Read the model definition and answer for the solid it produces. Units are mm, in the model's axes. Face numbers are marked on the shaded views. Round coordinates to 2 decimals unless told otherwise and drop trailing zeros. Loops run counter-clockwise (first coordinate to the right, second up) from the corner with the lowest first, then second, coordinate; pieces in that order, holes last. Notation, with made-up numbers: (-21, 64) - (25, 64) arc R22 cw to (25, 90) - close; hole circle Ø11 at (37.5, 41). An arc over 180 degrees is marked (long way). Answer as CSV lines item,"result".
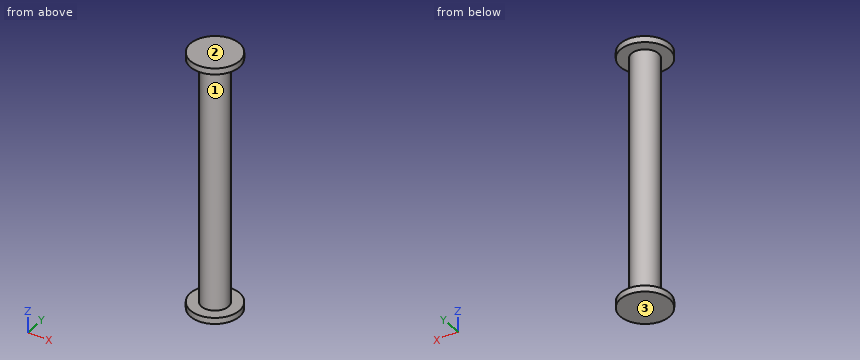
```python
from build123d import *

# Parameters (mm, degrees)
SKETCH1_R           = 2.2
BOSS_EXTRUDE1_DEPTH = 40
SKETCH2_R           = 4
BOSS_EXTRUDE2_DEPTH = 1
SKETCH3_R           = 4
BOSS_EXTRUDE3_DEPTH = 1


with BuildPart() as part:
    # Sketch1 → Boss-Extrude1 (new body)
    with BuildSketch(Plane.XY):
        with Locations((-44.111688034, 4.888301887)):
            Circle(SKETCH1_R)
    extrude(amount=-BOSS_EXTRUDE1_DEPTH)

    # Sketch2 → Boss-Extrude2 (add)
    with BuildSketch(Plane.XY):
        with Locations((-44.111688034, 4.888301887)):
            Circle(SKETCH2_R)
    extrude(amount=BOSS_EXTRUDE2_DEPTH)

    # Sketch3 → Boss-Extrude3 (add)
    with BuildSketch(Plane(origin=(0, 0, -40), x_dir=(-1, 0, 0), z_dir=(0, 0, -1))):
        with Locations((44.111688034, 4.888301887)):
            Circle(SKETCH3_R)
    extrude(amount=BOSS_EXTRUDE3_DEPTH)


solid = part.part
```
1) Each of these flat-tipped pins is pushed along its axis until it touches: P1, Ø2, axis at x = -46, z = -22.5, coming from the +Y side; P2, Ø3, axis at y = 4.5, z = -32.5, coming from the +X side; P3, Ø3, axis at y = 2.5, z = -27, coming from the -X side. Where does it stop, or does it pass through?
Entries:
P1,"stops at y = 6.9"
P2,"stops at x = -41.91"
P3,"stops at x = -46.12"
2) A cutting plane is placed at D-D, the plane x = -43.75. Determine the outline of the cut face in (y, z).
Entries:
outline,"(0.9, -41) - (8.87, -41) - (8.87, -40) - (7.06, -40) - (7.06, 0) - (8.87, 0) - (8.87, 1) - (0.9, 1) - (0.9, 0) - (2.72, 0) - (2.72, -40) - (0.9, -40) - close"
3) A cutting plane is placed at C-C, the plane y = 6.25. Determine the outline of the cut face in (x, z), plus the area to 3 significant figures.
Entries:
outline,"(-47.87, -41) - (-40.35, -41) - (-40.35, -40) - (-42.38, -40) - (-42.38, 0) - (-40.35, 0) - (-40.35, 1) - (-47.87, 1) - (-47.87, 0) - (-45.84, 0) - (-45.84, -40) - (-47.87, -40) - close"
area,"153 mm^2"
4) A cutting plane is placed at A-A, the plane x = -46.75. Determine the outline of the cut face in (y, z).
Entries:
outline,"(1.88, -41) - (7.89, -41) - (7.89, -40) - (1.88, -40) - close; (1.88, 0) - (7.89, 0) - (7.89, 1) - (1.88, 1) - close"
5) A cutting plane is placed at B-B, the plane y = 1.5. Determine the outline of the cut face in (x, z), plus the area to 3 significant figures.
Entries:
outline,"(-46.24, -41) - (-41.99, -41) - (-41.99, -40) - (-46.24, -40) - close; (-46.24, 0) - (-41.99, 0) - (-41.99, 1) - (-46.24, 1) - close"
area,"8.50 mm^2"
6) Find the intervals of material crossed by line 1 (Z direction, x = -45, y = 7.25); line 2 (X direction, y = 5, z = -14.5); line 3 (Y direction, x = -43.5, z = -18), in increasing order.
Entries:
line 1,"z = -41 to -40, 0 to 1"
line 2,"x = -46.31 to -41.91"
line 3,"y = 2.78 to 7"
7) The mould has two halves that part along Z. Classify the marked faces 1, 2 and 3: pulls with the +Z half, pulls with the -Z half, needs draft (parallel to the pull), parting line crosses it, or undercut.
Entries:
face 1,"undercut"
face 2,"pulls with the +Z half"
face 3,"pulls with the -Z half"
